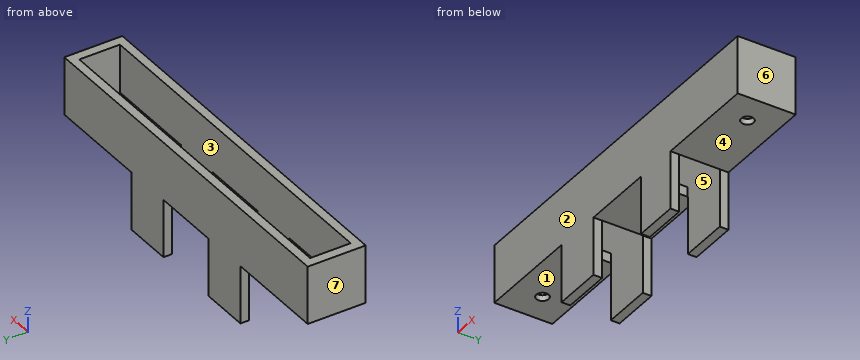
Autodesk Fusion 360 part; units mm, degrees
sketch "Sketch1" plane through (0, 0, 0) normal (0, 0, 1) x (1, 0, 0)
  line L0 (-18.2, 3) -> (78.32, 3)
  line L1 (78.32, 3) -> (78.32, -12)
  line L2 (78.32, -12) -> (-18.2, -12)
  line L3 (-18.2, -12) -> (-18.2, 3)
  line L4 (-18.2, 3) -> (8.47, 3)
  line L5 (8.47, 3) -> (8.47, 0.5)
  line L6 (8.47, 0.5) -> (21.12, 0.5)
  line L7 (21.12, 0.5) -> (21.12, 3)
  line L8 (78.32, 3) -> (51.65, 3)
  line L9 (51.65, 3) -> (39, 3)
  line L10 (39, 3) -> (39, 0.5)
  line L11 (39, 0.5) -> (51.65, 0.5)
  line L12 (51.65, 0.5) -> (51.65, 3)
  line L13 (8.47, -12) -> (21.12, -12)
  line L14 (8.47, -12) -> (8.47, -9.5)
  line L15 (8.47, -9.5) -> (21.12, -9.5)
  line L16 (21.12, -9.5) -> (21.12, -12)
  line L17 (51.65, -12) -> (39, -12)
  line L18 (40, -12) -> (40, -9.5)
  line L19 (51.65, -12) -> (51.65, -9.5)
  line L20 (40, -9.5) -> (51.65, -9.5)
  dimension "d1" = 96.52
  dimension "d2" = 15
  dimension "d3" = 26.67
  dimension "d4" = 2.5
  dimension "d5" = 12.65
  dimension "d6" = 26.67
  dimension "d7" = 12.65
  dimension "d8" = 12.65
  dimension "d9" = 2.5
  dimension "d10" = 12.65
  dimension "d11" = 2.5
  dimension "d12" = 2.5
extrude "Extrude1" add sketch "Sketch1" along normal blind 15 contours L0 L1 L2 L3 L4 L5 L6 L7 L8 L10 L11 L12 L14 L15 L16 L17 L18 L19 L20 makes body 1
sketch "Sketch2" plane through (0, 0, 0) normal (0, 0, -1) x (1, 0, 0)
  line L0 (40, 9.5) -> (40, 12)
  line L1 (40, 12) -> (21.12, 12)
  line L2 (21.12, 12) -> (21.12, 9.5)
  line L3 (21.12, 9.5) -> (8.47, 9.5)
  line L4 (8.47, 9.5) -> (8.47, 12)
  line L5 (8.47, 12) -> (-18.2, 12)
  line L6 (-18.2, 12) -> (-18.2, -3)
  line L7 (-18.2, -3) -> (8.47, -3)
  line L8 (8.47, -3) -> (8.47, -0.5)
  line L9 (8.47, -0.5) -> (21.12, -0.5)
  line L10 (21.12, -0.5) -> (21.12, -3)
  line L11 (21.12, -3) -> (39, -3)
  line L12 (39, -3) -> (39, -0.5)
  line L13 (39, -0.5) -> (51.65, -0.5)
  line L14 (51.65, -0.5) -> (51.65, -3)
  line L15 (51.65, -3) -> (78.32, -3)
  line L16 (78.32, -3) -> (78.32, 12)
  line L17 (78.32, 12) -> (51.65, 12)
  line L18 (51.65, 12) -> (51.65, 9.5)
  line L19 (51.65, 9.5) -> (40, 9.5)
  line L20 (8.47, 12) -> (21.12, 12)
  line L21 (21.12, 12) -> (21.12, 9.5)
  line L22 (21.12, 9.5) -> (8.47, 9.5)
  line L23 (8.47, 9.5) -> (8.47, 12)
  line L24 (8.47, -0.5) -> (21.12, -0.5)
  line L25 (21.12, -0.5) -> (21.12, -3)
  line L26 (21.12, -3) -> (8.47, -3)
  line L27 (8.47, -3) -> (8.47, -0.5)
  line L28 (40, 12) -> (51.65, 12)
  line L29 (51.65, 12) -> (51.65, 9.5)
  line L30 (51.65, 9.5) -> (40, 9.5)
  line L31 (40, 9.5) -> (40, 12)
  line L32 (39, -0.5) -> (51.65, -0.5)
  line L33 (51.65, -0.5) -> (51.65, -3)
  line L34 (51.65, -3) -> (39, -3)
  line L35 (39, -3) -> (39, -0.5)
extrude "Extrude2" add sketch "Sketch2" along normal blind 15 separate body contours L0 L18 L19 L28 L29 L30 L31 | L2 L3 L4 L20 L21 L22 L23 | L12 L13 L14 L32 L33 L34 L35 | L8 L9 L10 L24 L25 L26 L27 makes body 2 at (47.7667, -9.5, -5) makes body 3 at (47.4333, 3, -5) makes body 4 at (16.9033, -9.5, -5) makes body 5 at (12.6867, 0.5, -5)
extrude "Extrude3" add 4 faces at (43.2167, 1.3333, 0) (12.6867, 1.3333, 0) (16.9033, -11.1667, 0) (47.7667, -10.3333, 0) along direction (0, 0, 1) blind 15 on bodies 2 3 4 5 bodies 1 3 2 4 5
sketch "Sketch3" plane through (0, 0, 15) normal (0, 0, 1) x (-1, 0, 0)
  line L0 (18.2, 12) -> (-78.32, 12)
  line L1 (-78.32, 12) -> (-78.32, -3)
  line L2 (-78.32, -3) -> (18.2, -3)
  line L3 (18.2, -3) -> (18.2, 12)
  line L4 (-75.82, 9.75) -> (15.7, 9.75)
  line L5 (15.7, 9.75) -> (15.7, -0.75)
  line L6 (15.7, -0.75) -> (-75.82, -0.75)
  line L7 (-75.82, -0.75) -> (-75.82, 9.75)
  line L8 (-78.32, 12) -> (-75.82, 12)
  line L9 (-75.82, 12) -> (-75.82, 9.75)
  dimension "d19" = 91.52
  dimension "d20" = 10.5
  dimension "d21" = 2.5
  dimension "d22" = 2.25
extrude "Extrude4" cut sketch "Sketch3" against normal blind 12.5 contours L4 L5 L6 L7 bodies 1
sketch "Sketch4" plane through (0, 0, 2.5) normal (0, 0, 1) x (-1, 0, 0)
  line L0 (-75.82, -0.75) -> (15.7, -0.75)
  line L1 (15.7, -0.75) -> (15.7, 9.75)
  line L2 (15.7, 9.75) -> (-75.82, 9.75)
  line L3 (-75.82, 9.75) -> (-75.82, -0.75)
  line L4 (-75.82, 4.5) -> (-70.7, 4.5)
  circle A0 centre (-70.7, 4.5) radius 1.6
  line L5 (15.7, 4.5) -> (10.58, 4.5)
  circle A1 centre (10.58, 4.5) radius 1.6
  dimension "d25" = 5.12
  dimension "d26" = 3.2
  dimension "d27" = 5.12
  dimension "d28" = 3.2
extrude "Extrude5" cut sketch "Sketch4" against normal blind 100 contours A1 | A0 bodies 1
sketch "Sketch5" plane through (0, 0, 2.5) normal (0, 0, 1) x (-1, 0, 0)
  circle A0 centre (10.58, 4.5) radius 1.6
  circle A1 centre (-70.7, 4.5) radius 1.6
  line L0 (-75.82, -0.75) -> (15.7, -0.75)
  line L1 (15.7, -0.75) -> (15.7, 9.75)
  line L2 (15.7, 9.75) -> (-75.82, 9.75)
  line L3 (-75.82, 9.75) -> (-75.82, -0.75)
  circle A2 centre (10.58, 4.5) radius 3.5
  circle A3 centre (-70.7, 4.5) radius 3.5
  dimension "d31" = 7
  dimension "d32" = 7
extrude "Extrude6" cut sketch "Sketch5" against normal blind 1 contours A2 | A3 bodies 1
sketch "Sketch6" plane through (0, 0, 2.5) normal (0, 0, 1) x (-1, 0, 0)
  circle A0 centre (-70.7, 4.5) radius 3.5
  circle A1 centre (10.58, 4.5) radius 3.5
  line L0 (-75.82, -0.75) -> (15.7, -0.75)
  line L1 (15.7, -0.75) -> (15.7, 9.75)
  line L2 (15.7, 9.75) -> (-75.82, 9.75)
  line L3 (-75.82, 9.75) -> (-75.82, -0.75)
  line L4 (-75.82, 4.5) -> (-78.3, 4.5)
  line L5 (-75.82, 4.5) -> (-51.65, 4.5)
  line L6 (-51.65, 4.5) -> (-38.95, 4.5)
  line L7 (15.7, 4.5) -> (-8.47, 4.5)
  line L8 (-8.47, 4.5) -> (-21.17, 4.5)
  line L9 (-38.95, 9.75) -> (-51.65, 9.75)
  line L10 (-51.65, 9.75) -> (-51.65, -0.75)
  line L11 (-51.65, -0.75) -> (-38.95, -0.75)
  line L12 (-38.95, -0.75) -> (-38.95, 9.75)
  line L13 (-8.47, -0.75) -> (-21.17, -0.75)
  line L14 (-21.17, -0.75) -> (-21.17, 9.75)
  line L15 (-21.17, 9.75) -> (-8.47, 9.75)
  line L16 (-8.47, 9.75) -> (-8.47, -0.75)
  dimension "d35" = 24.17
  dimension "d36" = 12.7
  dimension "d37" = 24.17
  dimension "d38" = 12.7
extrude "Extrude7" cut sketch "Sketch6" against normal blind 100 contours L2 L6 L9 L10 L12 | L0 L6 L10 L11 L12 | L0 L8 L13 L14 L16 | L2 L8 L14 L15 L16 bodies 1
Verification items for the finished model (mm, model axes). Face numbers are marked on the shaded views. A direction names the side the tool comes from. Coordinates: 2 decimals unless noted, no trailing zeros. Write each loop counter-clockwise with the first axis right and the second up, starting at its lowest first coordinate (ties: lowest second). Pieces come first, ordered by that corner, then holes. Notation, with made-up numbers: M 44,62.25 L 67,62.25 A31 ccw 67,101.25 Z; hole C 61.5,33.25 d6. An arc over 180 degrees is marked long. One line per item, written item: value.
Item 1: Gauge pin test, flat ends, axial feed: pin 1 Ø1.1 at (y, z) = (2, -11) entering from +X; pin 2 Ø8 at (x, y) = (2, -3.5) entering from -Z; pin 3 Ø2 at (y, z) = (-1, -6) entering from -X; pin 4 Ø3.5 at (x, y) = (70.7, -4.5) entering from +Z. Record the tip position at first contact, or that the pin passes through.
Check sheet entries:
pin 1: stops at x = 51.65
pin 2: stops at z = 0
pin 3: passes through
pin 4: stops at z = 1.5
Item 2: Mould release check, pull along X, two halves, no side actions. Record for the marked faces 4, 5, 6 and 7: pulls with the +X half, pulls with the -X half, needs draft (parallel to the pull), parting line crosses it, or undercut.
Check sheet entries:
face 4: needs draft
face 5: undercut
face 6: pulls with the +X half
face 7: pulls with the -X half
Item 3: Section check A-A, the plane y = -4.5. State how many separate pieces and enclosed holes the cut face has, plus the area to 3 significant figures.
Check sheet entries:
separate pieces: 5
enclosed holes: 0
area: 217 mm^2
Item 4: Section check C-C, the plane z = -13. Record the boundary of the cut face in (x, y).
Check sheet entries:
outline: M 8.47,-12 L 21.12,-12 L 21.12,-9.75 L 8.47,-9.75 Z; M 8.47,0.75 L 21.12,0.75 L 21.12,3 L 8.47,3 Z; M 39,0.75 L 51.65,0.75 L 51.65,3 L 39,3 Z; M 40,-12 L 51.65,-12 L 51.65,-9.75 L 40,-9.75 Z
Item 5: Access from +Z, -Z, +X, -X, +Y, -Y to the whole of each face (thin tool, end or side, straight path). Record for the marked faces 1, 2 and 3.
Check sheet entries:
face 1: -Z, -X, +Y, -Y
face 2: +Z, -Z, +X, -X, -Y
face 3: +Z
Item 6: Section check B-B, the plane x = 49. Record the boundary of the cut face in (y, z), plus the area to 3 significant figures.
Check sheet entries:
outline: M -12,-15 L -9.75,-15 L -9.75,15 L -12,15 Z; M 0.75,-15 L 3,-15 L 3,15 L 0.75,15 Z
area: 135 mm^2
Item 7: Scan lines: line 1 along X through (y, z) = (-4.5, 1.1); line 2 along X through (y, z) = (-4.5, 2); line 3 along X through (y, z) = (2.5, -10). Record each from-to range of solid material in increasing order.
Check sheet entries:
line 1: x = -18.2 to -12.18, -8.98 to 8.47, 21.17 to 38.95, 51.65 to 69.1, 72.3 to 78.32
line 2: x = -18.2 to -14.08, -7.08 to 8.47, 21.17 to 38.95, 51.65 to 67.2, 74.2 to 78.32
line 3: x = 8.47 to 21.12, 39 to 51.65
Item 8: Section check D-D, the plane z = 12. Record the boundary of the cut face in (x, y), plus the area to 3 significant figures.
Check sheet entries:
outline: M -18.2,-12 L 78.32,-12 L 78.32,3 L -18.2,3 Z; hole M -15.7,-9.75 L 75.82,-9.75 L 75.82,0.75 L -15.7,0.75 Z
area: 487 mm^2
